For this review, take the finished solid that the model builds, in its own axes (mm). Face numbers are marked on the shaded views. Round coordinates to 2 decimals unless told otherwise and drop trailing zeros. Write each loop counter-clockwise with the first axis right and the second up, starting at its lowest first coordinate (ties: lowest second). Pieces come first, ordered by that corner, then holes. Notation, with made-up numbers: (-9.75, -12.5) -> (40.25, -12.5) arc R25 cw to (40.25, 3.5) -> close; hole circle Ø9 at (-5, -24.75). An arc over 180 degrees is marked (long way). Answer as CSV lines item,"result". Start each with the question number.
Item 1: Wall thickness on probe 1 along Z at (x, y) = (-83.5, 5); probe 2 along Z at (x, y) = (-128.5, 7); probe 3 along X at (y, z) = (-7, -105): over which ranges is each line inside the solid? List them lowest first. Write a range as from..to.
Item 2: For pin 1 Ø10 at (x, y) = (-165.5, -3.5) entering from +Z; pin 2 Ø12 at (x, y) = (-139.5, 14.5) entering from -Z; pin 3 Ø8 at (x, y) = (-48, 7.5) entering from -Z, all flat-tipped, find the tip position at first contact; note any pin that passes through.
Item 3: Take a section at C-C on x = -197.5. Give the boundary of the cut face in (y, z).
Item 4: Take a section at B-B on z = -34. Give the boundary of the cut face in (x, y).
Item 5: Take a section at D-D on z = -233. Give the boundary of the cut face in (x, y).
Item 6: Take a section at A-A on x = -43. Give the boundary of the cut face in (y, z), then the cut area to 3 significant figures.
Item 7: Mouldability with a two-part tool opening along Z and no side actions: class the marked faces 1 and 2 as +Z half, -Z half, draft (parallel to the pull), parting line (faces both ways), or undercut.
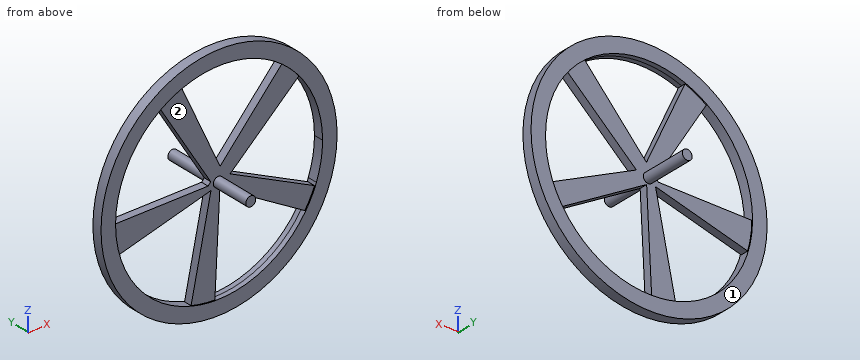
```python
from build123d import *

# Parameters (mm, degrees)
F0_R     = 300
F1_DEPTH = 12.5
F2_DEPTH = 10
F3_R     = 12.5
F4_DEPTH = 120


with BuildPart() as f1:
    # F0 (on Front) → F1 (new body, symmetric)
    with BuildSketch(Plane.XZ):
        Circle(F0_R)
        with BuildLine():
            ThreePointArc((205.0956009639, 164.7581922724), (248.1586056274, 87.3314027639), (263.0769230769, 0))
            ThreePointArc((263.0769230769, 0), (259.1250629437, -45.4276260667), (247.3882097841, -89.4904526497))
            Line((247.3882097841, -89.4904526497), (253.5845122853, -126.7404960598))
            Line((253.5845122853, -126.7404960598), (220.0723785431, -144.1444263855))
            ThreePointArc((220.0723785431, -144.1444263855), (121.2485164836, -233.4700509833), (-8.6633171075, -262.9342396728))
            Line((-8.6633171075, -262.9342396728), (-42.1754508497, -280.3381699985))
            Line((-42.1754508497, -280.3381699985), (-69.0833910393, -253.8443470675))
            ThreePointArc((-69.0833910393, -253.8443470675), (-184.5753612112, -187.4604051243), (-252.7424342118, -73.0118442742))
            Line((-252.7424342118, -73.0118442742), (-279.6503744013, -46.5180213432))
            Line((-279.6503744013, -46.5180213432), (-263.0769230769, 0))
            ThreePointArc((-263.0769230769, 0), (-232.4046711792, 123.2782879087), (-147.5400976348, 217.8104383301))
            Line((-147.5400976348, 217.8104383301), (-130.6579854969, 251.588451719))
            Line((-130.6579854969, 251.588451719), (-93.3163262043, 245.9705891349))
            ThreePointArc((-93.3163262043, 245.9705891349), (39.138142442, 260.1493287745), (161.55763917, 207.6260982667))
            Line((161.55763917, 207.6260982667), (198.8992984626, 202.0082356825))
            Line((198.8992984626, 202.0082356825), (205.0956009639, 164.7581922724))
        make_face(mode=Mode.SUBTRACT)
        with BuildLine():
            ThreePointArc((-147.5400976348, 217.8104383301), (-121.2485164836, 233.4700509833), (-93.3163262043, 245.9705891349))
            Line((-93.3163262043, 245.9705891349), (-130.6579854969, 251.588451719))
            Line((-130.6579854969, 251.588451719), (-147.5400976348, 217.8104383301))
        make_face()
        with BuildLine():
            ThreePointArc((-252.7424342118, -73.0118442742), (-260.4804881167, -36.8698083275), (-263.0769230769, 0))
            Line((-263.0769230769, 0), (-279.6503744013, -46.5180213432))
            Line((-279.6503744013, -46.5180213432), (-252.7424342118, -73.0118442742))
        make_face()
        with BuildLine():
            Line((-42.1754508497, -280.3381699985), (-8.6633171075, -262.9342396728))
            ThreePointArc((-8.6633171075, -262.9342396728), (-39.138142442, -260.1493287745), (-69.0833910393, -253.8443470675))
            Line((-69.0833910393, -253.8443470675), (-42.1754508497, -280.3381699985))
        make_face()
        with BuildLine():
            Line((253.5845122853, -126.7404960598), (247.3882097841, -89.4904526497))
            ThreePointArc((247.3882097841, -89.4904526497), (246.0347091348, -93.1471382093), (244.6271617936, -96.7833620434))
            ThreePointArc((244.6271617936, -96.7833620434), (233.553384264, -121.0879191102), (220.0723785431, -144.1444263855))
            Line((220.0723785431, -144.1444263855), (253.5845122853, -126.7404960598))
        make_face()
        with BuildLine():
            ThreePointArc((161.55763917, 207.6260982667), (184.5753612112, 187.4604051243), (205.0956009639, 164.7581922724))
            Line((205.0956009639, 164.7581922724), (198.8992984626, 202.0082356825))
            Line((198.8992984626, 202.0082356825), (161.55763917, 207.6260982667))
        make_face()
    extrude(amount=F1_DEPTH, both=True)

    # F0 (on Front) → F2 (join, symmetric)
    with BuildSketch(Plane.XZ):
        with BuildLine():
            Line((244.6271617936, -96.7833620434), (30.1419629049, 7.3265620085))
            Line((30.1419629049, 7.3265620085), (12.8380831788, 15.7257691026))
            Line((12.8380831788, 15.7257691026), (4.5759868907, 33.6459373179))
            Line((4.5759868907, 33.6459373179), (-93.3163262043, 245.9705891349))
            ThreePointArc((-93.3163262043, 245.9705891349), (-121.2485164836, 233.4700509833), (-147.5400976348, 217.8104383301))
            Line((-147.5400976348, 217.8104383301), (-19.0782173139, 7.4303752131))
            Line((-19.0782173139, 7.4303752131), (-25.7826172389, 0))
            Line((-25.7826172389, 0), (-263.0769230769, 0))
            ThreePointArc((-263.0769230769, 0), (-260.4804881167, -36.8698083275), (-252.7424342118, -73.0118442742))
            Line((-252.7424342118, -73.0118442742), (-18.4854909648, -12.6607832838))
            Line((-18.4854909649, -12.6607832838), (-69.0833910393, -253.8443470675))
            ThreePointArc((-69.0833910393, -253.8443470675), (-39.138142442, -260.1493287745), (-8.6633171075, -262.9342396728))
            Line((-8.6633171075, -262.9342396728), (4.1106084022, -16.0976926844))
            Line((4.1106084022, -16.0976926844), (220.0723785431, -144.1444263855))
            ThreePointArc((220.0723785431, -144.1444263855), (233.553384264, -121.0879191102), (244.6271617936, -96.7833620434))
        make_face()
        with BuildLine():
            Line((30.1419629049, 7.3265620085), (205.0956009639, 164.7581922724))
            ThreePointArc((205.0956009639, 164.7581922724), (184.5753612112, 187.4604051243), (161.55763917, 207.6260982667))
            Line((161.55763917, 207.6260982667), (4.5759868907, 33.6459373179))
            Line((4.5759868907, 33.6459373179), (12.8380831788, 15.7257691026))
            Line((12.8380831788, 15.7257691026), (30.1419629049, 7.3265620085))
        make_face()
    extrude(amount=F2_DEPTH, both=True)

    # F3 (on face) → F4 (join, symmetric)
    with BuildSketch(Plane(origin=(0, 10, 0), x_dir=(-1, 0, 0), z_dir=(0, 1, 0))):
        Circle(F3_R)
    extrude(amount=F4_DEPTH, both=True)


solid = f1.part
```
Output values:
1,probe 1,"z = -288.15..-249.47, -29.41..0, 112.93..224.68, 249.47..288.15"
1,probe 2,"z = -271.09..-229.56, -41..0, 186.63..271.09"
1,probe 3,"x = -281.02..-241.21, -37.86..-0.49, 154.05..281.02"
2,pin 1,"stops at z = 253.46"
2,pin 2,"stops at z = -268.49"
2,pin 3,"stops at z = -296.76"
3,outline,"(-12.5, -225.82) -> (12.5, -225.82) -> (12.5, -173.79) -> (-12.5, -173.79) -> close; (-12.5, 173.79) -> (12.5, 173.79) -> (12.5, 225.82) -> (-12.5, 225.82) -> close; (-10, -58.78) -> (10, -58.78) -> (10, 0) -> (-10, 0) -> close"
4,outline,"(-298.07, -12.5) -> (-260.87, -12.5) -> (-260.87, -10) -> (-101.32, -10) -> (-101.32, 10) -> (-260.87, 10) -> (-260.87, 12.5) -> (-298.07, 12.5) -> close; (-22.96, -10) -> (3.18, -10) -> (3.18, 10) -> (-22.96, 10) -> close; (34.3, -10) -> (115.28, -10) -> (115.28, 10) -> (34.3, 10) -> close; (260.87, -12.5) -> (298.07, -12.5) -> (298.07, 12.5) -> (260.87, 12.5) -> close"
5,outline,"(-188.97, -12.5) -> (-122.15, -12.5) -> (-122.15, 12.5) -> (-188.97, 12.5) -> close; (-64.71, -10) -> (-7.11, -10) -> (-7.11, 10) -> (-64.71, 10) -> close; (122.15, -12.5) -> (188.97, -12.5) -> (188.97, 12.5) -> (122.15, 12.5) -> close"
6,outline,"(-12.5, -296.9) -> (12.5, -296.9) -> (12.5, -259.54) -> (10, -259.54) -> (10, -129.51) -> (-10, -129.51) -> (-10, -259.54) -> (-12.5, -259.54) -> close; (-12.5, 259.54) -> (12.5, 259.54) -> (12.5, 296.9) -> (-12.5, 296.9) -> close; (-10, -18.98) -> (10, -18.98) -> (10, 0) -> (-10, 0) -> close; (-10, 46.61) -> (10, 46.61) -> (10, 136.84) -> (-10, 136.84) -> close"
6,area,"6,650 mm^2"
7,face 1,"draft"
7,face 2,"undercut"
